Input: part model. Units: mm. Frame: model coordinates. A direction names the side the tool comes from. Coordinates: 2 decimals unless noted, no trailing zeros. Write each loop counter-clockwise with the first axis right and the second up, starting at its lowest first coordinate (ties: lowest second). Pieces come first, ordered by that corner, then holes.
from build123d import *

# Parameters (mm, degrees)
F0_R      = 52.07
F1_DEPTH  = 5.08
F0_R_2    = 55.245
F2_DEPTH  = 30.48
F4_DEPTH  = 21.59
F5_W      = 9.2520020868
F5_H      = 19.05
F6_DEPTH  = 50.8
F7_W      = 9.2520020868
F7_H      = 19.05
F8_DEPTH  = 50.8
F9_W      = 9.2520020868
F9_H      = 19.05
F10_DEPTH = 50.8
F11_W     = 19.05
F11_H     = 9.2520020868
F12_DEPTH = 50.8
F13_W     = 19.05
F13_H     = 9.2520020868
F14_DEPTH = 50.8
F15_W     = 19.05
F15_H     = 9.2520020868
F16_DEPTH = 50.8
F17_W     = 9.2520020868
F17_H     = 19.05
F18_DEPTH = 50.8
F19_W     = 9.2520020868
F19_H     = 19.05
F20_DEPTH = 50.8
F21_W     = 9.2520020868
F21_H     = 19.05
F22_DEPTH = 50.8
F23_W     = 19.05
F23_H     = 9.2520020868
F24_DEPTH = 50.8
F25_W     = 19.05
F25_H     = 9.2520020868
F26_DEPTH = 50.8
F27_W     = 19.05
F27_H     = 9.2520020868
F28_DEPTH = 50.8
F29_DEPTH = 21.59
F30_R     = 2.9464
F31_DEPTH = 8.382


with BuildPart() as f1:
    # F0 (on Front) → F1 (new body)
    with BuildSketch(Plane.XZ):
        Circle(F0_R)
    extrude(amount=F1_DEPTH)

    # F0 (on Front) → F2 (join)
    with BuildSketch(Plane.XZ):
        Circle(F0_R_2)
        Circle(F0_R, mode=Mode.SUBTRACT)
    extrude(amount=F2_DEPTH)

    # F3 (on face) → F4 (join)
    with BuildSketch(Plane.XZ.offset(5.08)):
        Polygon((4.5521322669, -17.2840948262), (12.5843095976, -12.6923990675), (17.2445313344, -4.6997852286), (17.2840948262, 4.5521322669), (12.6923990675, 12.5843095976), (4.6997852286, 17.2445313344), (-4.5521322669, 17.2840948262), (-12.5843095976, 12.6923990675), (-17.2445313344, 4.6997852286), (-17.2840948262, -4.5521322669), (-12.6923990675, -12.5843095976), (-4.6997852286, -17.2445313344), align=None)
    extrude(amount=F4_DEPTH)

    # F5 (on face) → F6 (cut)
    with BuildSketch(Plane(origin=(8.696092148, 0, 14.914420466), x_dir=(0.8638793813, 0, -0.5036987339), z_dir=(0.5036987339, 0, 0.8638793813))):
        with Locations((0, -17.145)):
            Rectangle(F5_W, F5_H)
    extrude(amount=F6_DEPTH, mode=Mode.SUBTRACT)

    # F7 (on face) → F8 (cut)
    with BuildSketch(Plane(origin=(0.0738264808, 0, 17.2643130803), x_dir=(0.999990857, 0, -0.0042762087), z_dir=(0.0042762087, 0, 0.999990857))):
        with Locations((0, -17.145)):
            Rectangle(F7_W, F7_H)
    extrude(amount=F8_DEPTH, mode=Mode.SUBTRACT)

    # F9 (on face) → F10 (cut)
    with BuildSketch(Plane(origin=(-8.5682209323, 0, 14.9882469469), x_dir=(0.86815559, 0, 0.4962921231), z_dir=(-0.4962921231, 0, 0.86815559))):
        with Locations((0, -17.145)):
            Rectangle(F9_W, F9_H)
    extrude(amount=F10_DEPTH, mode=Mode.SUBTRACT)

    # F11 (on face) → F12 (cut)
    with BuildSketch(Plane(origin=(-14.914420466, 0, 8.696092148), x_dir=(0, -1, 0), z_dir=(-0.8638793813, 0, 0.5036987339))):
        with Locations((17.145, 0)):
            Rectangle(F11_W, F11_H)
    extrude(amount=F12_DEPTH, mode=Mode.SUBTRACT)

    # F13 (on face) → F14 (cut)
    with BuildSketch(Plane(origin=(-17.2643130803, 0, 0.0738264808), x_dir=(0, -1, 0), z_dir=(-0.999990857, 0, 0.0042762087))):
        with Locations((17.145, 0)):
            Rectangle(F13_W, F13_H)
    extrude(amount=F14_DEPTH, mode=Mode.SUBTRACT)

    # F15 (on face) → F16 (cut)
    with BuildSketch(Plane(origin=(-14.9882469469, 0, -8.5682209323), x_dir=(0, -1, 0), z_dir=(-0.86815559, 0, -0.4962921231))):
        with Locations((17.145, 0)):
            Rectangle(F15_W, F15_H)
    extrude(amount=F16_DEPTH, mode=Mode.SUBTRACT)

    # F17 (on face) → F18 (cut)
    with BuildSketch(Plane(origin=(-8.696092148, 0, -14.914420466), x_dir=(0.8638793813, 0, -0.5036987339), z_dir=(-0.5036987339, 0, -0.8638793813))):
        with Locations((0, 17.145)):
            Rectangle(F17_W, F17_H)
    extrude(amount=F18_DEPTH, mode=Mode.SUBTRACT)

    # F19 (on face) → F20 (cut)
    with BuildSketch(Plane(origin=(-0.0738264808, 0, -17.2643130803), x_dir=(0.999990857, 0, -0.0042762087), z_dir=(-0.0042762087, 0, -0.999990857))):
        with Locations((0, 17.145)):
            Rectangle(F19_W, F19_H)
    extrude(amount=F20_DEPTH, mode=Mode.SUBTRACT)

    # F21 (on face) → F22 (cut)
    with BuildSketch(Plane(origin=(8.5682209323, 0, -14.9882469469), x_dir=(0.86815559, 0, 0.4962921231), z_dir=(0.4962921231, 0, -0.86815559))):
        with Locations((0, 17.145)):
            Rectangle(F21_W, F21_H)
    extrude(amount=F22_DEPTH, mode=Mode.SUBTRACT)

    # F23 (on face) → F24 (cut)
    with BuildSketch(Plane(origin=(14.914420466, 0, -8.696092148), x_dir=(0, 1, 0), z_dir=(0.8638793813, 0, -0.5036987339))):
        with Locations((-17.145, 0)):
            Rectangle(F23_W, F23_H)
    extrude(amount=F24_DEPTH, mode=Mode.SUBTRACT)

    # F25 (on face) → F26 (cut)
    with BuildSketch(Plane(origin=(17.2643130803, 0, -0.0738264808), x_dir=(0, 1, 0), z_dir=(0.999990857, 0, -0.0042762087))):
        with Locations((-17.145, 0)):
            Rectangle(F25_W, F25_H)
    extrude(amount=F26_DEPTH, mode=Mode.SUBTRACT)

    # F27 (on face) → F28 (cut)
    with BuildSketch(Plane(origin=(14.9882469469, 0, 8.5682209323), x_dir=(0, 1, 0), z_dir=(0.86815559, 0, 0.4962921231))):
        with Locations((-17.145, 0)):
            Rectangle(F27_W, F27_H)
    extrude(amount=F28_DEPTH, mode=Mode.SUBTRACT)

    # F29 (cut): a face of the model
    f29_faces = [f1.faces().sort_by_distance(p)[0] for p in [
        (0, -26.67, 0),
    ]]
    extrude(f29_faces, amount=-F29_DEPTH, mode=Mode.SUBTRACT)

    # F30 (on face) → F31 (cut)
    with BuildSketch(Plane.XZ.offset(5.08)):
        Circle(F30_R)
    extrude(amount=-F31_DEPTH, mode=Mode.SUBTRACT)


solid = f1.part
Item 1: Section query C-C, the plane y = -28. Return loops of the section in (x, z) (3 decimals), then the cut area to 3 significant figures.
Item 2: Pull-direction query (Y, two-part tool) for faces 5 (the face through (-1, 0, -12)), 6 (the face through (11, -5.08, 1)), 7 (the face through (54, -7.62, 0)); classes: released by +Y, released by -Y, zero draft, split by the parting line, or undercut.
Item 3: Section query A-A, the plane z = 0. Return loops of the section in (x, y) (3 decimals).
Item 4: Section query D-D, the plane x = 36. Return loops of the section in (y, z).
Item 5: Section query B-B, the plane x = 0. Return loops of the section in (y, z) (3 decimals).
Item 6: Pin query (flat end, axial travel): pin 1 Ø5 at (y, z) = (-6, -16.5) entering from +X; pin 2 Ø1.5 at (x, y) = (-33, -20.5) entering from -Z; pin 3 Ø3 at (y, z) = (-20.5, 41) entering from -X. Return the tip coordinate at first contact, or that it passes through.
Item 7: Material intervals for line 1 (Z direction, x = 0, y = -3.1) (3 decimals); line 2 (X direction, y = -12.5, z = -14); line 3 (X direction, y = -10, z = -6), sorted ascending.
Item 8: Access query for faces 1 (the face through (30.536, -17.012, -44.094)), 2 (the face through (-30.536, -17.278, 44.094)), 3 (the face through (22.503, -17.012, -48.686)), 4 (the face through (-11.98, -15.03, -53.93)). Directions: +Z, -Z, +X, -X, +Y, -Y. A direction counts if a zero-diameter tool reaches every point of the face in a straight line with its end or side. Return the directions, or none.
The answers:
1. outline: circle Ø110.49 at (0, 0); hole circle Ø104.14 at (0, 0)
1. area: 1,070 mm2
2. face 5: released by +Y
2. face 6: released by -Y
2. face 7: undercut
3. outline: (-55.245, -30.48) - (-52.07, -30.48) - (-52.07, -26.67) - (-55.245, -26.67) - close; (-55.245, -7.62) - (-52.07, -7.62) - (-52.07, -5.08) - (-2.946, -5.08) - (-2.946, 0) - (-55.245, 0) - close; (2.946, -5.08) - (52.07, -5.08) - (52.07, -7.62) - (55.245, -7.62) - (55.245, 0) - (2.946, 0) - close; (52.07, -30.48) - (55.245, -30.48) - (55.245, -26.67) - (52.07, -26.67) - close
4. outline: (-30.48, -41.9) - (0, -41.9) - (0, 41.9) - (-30.48, 41.9) - (-30.48, 37.62) - (-5.08, 37.62) - (-5.08, -37.62) - (-30.48, -37.62) - close
5. outline: (-30.48, -55.245) - (-26.67, -55.245) - (-26.67, -52.07) - (-30.48, -52.07) - close; (-30.48, 52.07) - (-26.67, 52.07) - (-26.67, 55.245) - (-30.48, 55.245) - close; (-7.62, -55.245) - (0, -55.245) - (0, -2.946) - (-5.08, -2.946) - (-5.08, -52.07) - (-7.62, -52.07) - close; (-7.62, 52.07) - (-5.08, 52.07) - (-5.08, 2.946) - (0, 2.946) - (0, 55.245) - (-7.62, 55.245) - close
6. pin 1: stops at x = 53.44
6. pin 2: stops at z = -44.85
6. pin 3: stops at x = -38.62
7. line 1: z = -55.245 to -2.946, 2.946 to 55.245
7. line 2: x = -53.44 to -50.15, 50.15 to 53.44
7. line 3: x = -54.92 to -51.72, 51.72 to 54.92
8. face 1: -Z
8. face 2: +Z
8. face 3: +X
8. face 4: +Y, -Y
